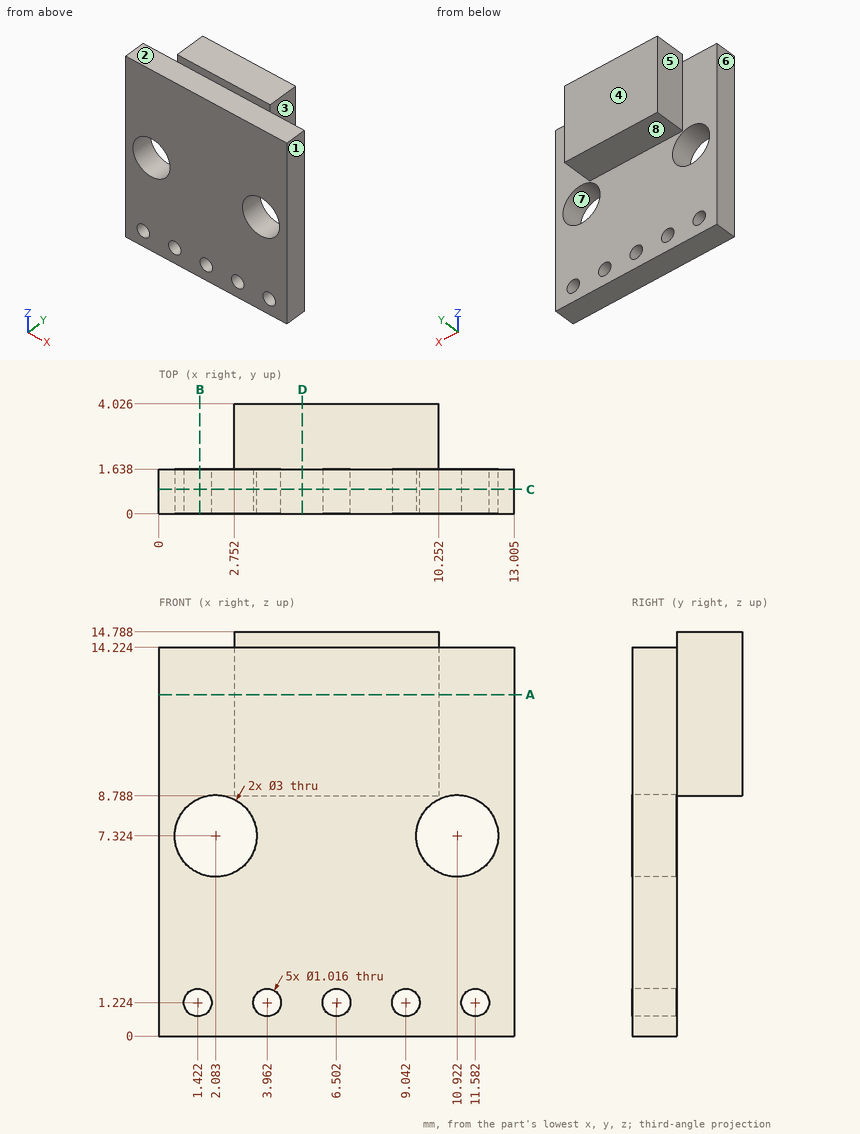
The figure shows three views and two pictorial views of one solid part (mm, origin at its lowest corner). Answer the questions. A direction names the side the tool comes from. Coordinates: 2 decimals unless noted, no trailing zeros. Order: outer loops, then holes, each group sorted by start corner. A loop starts at its lowest first (then second) coordinate and runs counter-clockwise, first axis right, second up.
Q1. A cutting plane is placed at D-D, the plane x = 5.25. Write down the section's boundary in (y, z).
Q2. A cutting plane is placed at C-C, the plane y = 0.9. State how many separate pieces and enclosed holes the cut face has, and give its area (3 significant figures).
Q3. A cutting plane is placed at B-B, the plane x = 1.5. Write down the section's boundary in (y, z).
Q4. Which of the six approach directions +Z, -Z, +X, -X, +Y, -Y give full straight-line access (tool end or side, diameter ignored) to the marked faces 1, 2, 3, 4 and 5?
Q5. For a pull along Z with two mould halves and no side action, classify the marked faces 6, 7 and 8 as pulls with the +Z half, pulls with the -Z half, needs draft (parallel to the pull), parting line crosses it, or undercut.
Q6. Consider line 1 (Z direction, x = 11.5, y = 0.3) (1 decimal); line 2 (X direction, y = 0.7, z = 6.25) (1 decimal); line 3 (Z direction, x = 5, y = 0.7). Determine where each line is inside the solid, lowest interval first.
Q7. A cutting plane is placed at A-A, the plane z = 12.5. Write down the section's boundary in (x, y) (1 decimal).
Q8. Given P1, Ø1.2, axis at y = 2.5, z = 13, coming from the -X side; P2, Ø1.3, axis at x = 9, y = 0.5, coming from the +Z side; P3, Ø1.6, axis at x = 9.04, z = 1.22, coming from the +Y side, each flat-ended and moving along its own axis, determine where each tip first touches the part or whether it passes through.
Answers follow:
1. outline: (0, 0) - (1.64, 0) - (1.64, 8.79) - (4.03, 8.79) - (4.03, 14.79) - (1.64, 14.79) - (1.64, 14.22) - (0, 14.22) - close
2. separate pieces: 1
2. enclosed holes: 7
2. area: 167 mm2
3. outline: (0, 0) - (1.64, 0) - (1.64, 0.72) - (0, 0.72) - close; (0, 1.73) - (1.64, 1.73) - (1.64, 5.94) - (0, 5.94) - close; (0, 8.71) - (1.64, 8.71) - (1.64, 14.22) - (0, 14.22) - close
4. face 1: +Z, -Z, +X, +Y, -Y
4. face 2: +Z, +X, -X, -Y
4. face 3: +Z, -Z, +X, +Y
4. face 4: +Z, -Z, +X, -X, +Y
4. face 5: +Z, -Z, -X, +Y
5. face 6: needs draft
5. face 7: undercut
5. face 8: pulls with the -Z half
6. line 1: z = 0 to 0.7, 1.7 to 5.9, 8.7 to 14.2
6. line 2: x = 0 to 1, 3.1 to 9.9, 12 to 13
6. line 3: z = 0 to 14.22
7. outline: (0, 0) - (13, 0) - (13, 1.6) - (10.3, 1.6) - (10.3, 4) - (2.8, 4) - (2.8, 1.6) - (0, 1.6) - close
8. P1: stops at x = 2.75
8. P2: stops at z = 14.22
8. P3: stops at y = 1.64
